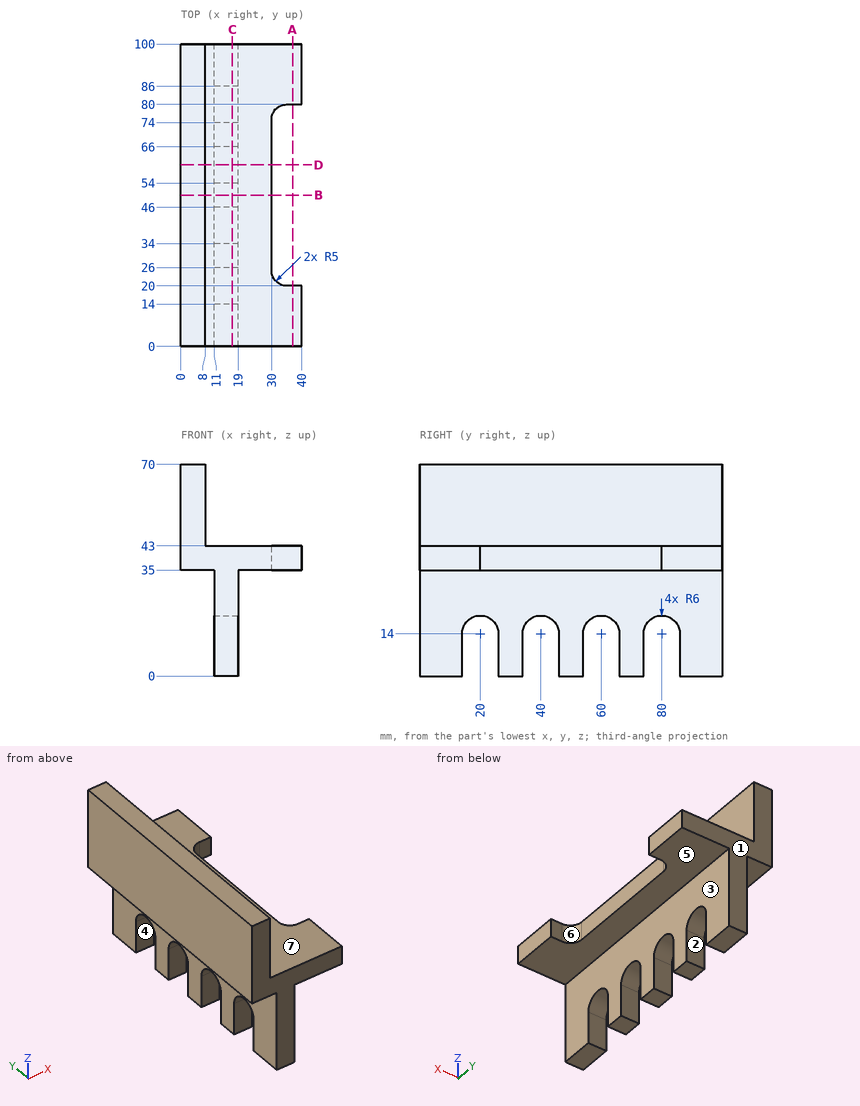
The figure shows three views and two pictorial views of one solid part (mm, origin at its lowest corner). Answer the questions. A direction names the side the tool comes from. Round coordinates to 2 decimals unless told otherwise and drop trailing zeros. Loops run counter-clockwise (first coordinate to the right, second up) from the corner with the lowest first, then second, coordinate; pieces in that order, holes last. Notation, with made-up numbers: M 24.5,27.5 L 38.5,27.5 A17 cw 38.5,48.5 Z; hole C 18.25,-15.5 d11. An arc over 180 degrees is marked long. Use CSV: the item, a comma, the result in double quotes.
Q1. The mould has two halves that part along Y. Classify the marked faces 1, 2 and 3: pulls with the +Y half, pulls with the -Y half, needs draft (parallel to the pull), parting line crosses it, or undercut.
Determined:
face 1,"pulls with the +Y half"
face 2,"undercut"
face 3,"needs draft"
Q2. Each of these flat-tipped pins is pushed along its axis until it touches: pin 1 (1 mm diameter, centred on x = 29.5, z = 42, fed in from -Y); pin 2 (8 mm diameter, centred on x = 24.5, y = 56.5, fed in from +Z); pin 3 (2.5 mm diameter, centred on y = 42.5, z = 40, fed in from +X); pin 4 (4 mm diameter, centred on y = 45, z = 49.5, fed in from +X). Where does it stop, or does it pass through?
Determined:
pin 1,"y = 0"
pin 2,"z = 43"
pin 3,"x = 30"
pin 4,"x = 8"
Q3. Section C-C, the plane x = 17 is taken. Determine the outline of the cut face in (y, z), then the cut area to 3 significant figures.
Determined:
outline,"M 0,0 L 14,0 L 14,14 A6 cw 26,14 L 26,0 L 34,0 L 34,14 A6 cw 46,14 L 46,0 L 54,0 L 54,14 A6 cw 66,14 L 66,0 L 74,0 L 74,14 A6 cw 86,14 L 86,0 L 100,0 L 100,43 L 0,43 Z"
area,"3,400 mm2"
Q4. A tool of negligible diameter and unlimited length cuts with its end or side. For the marked faces 4, 5, 6 and 7, from which of +Z, -Z, +X, -X, +Y, -Y can it reach the whole face along a straight path? Write none if from no direction.
Determined:
face 4,"-Z, +X, -X"
face 5,"-Z, +X, +Y, -Y"
face 6,"+Z, -Z, +X"
face 7,"+Z, +X, +Y, -Y"
Q5. Consider L1, parallel to Z at x = 2, y = 64; L2, parallel to Z at x = 36, y = 81; L3, parallel to X at y = 38, z = 56.5. Determine where each line is inside the solid, lowest interval first.
Determined:
L1,"35 to 70"
L2,"35 to 43"
L3,"0 to 8"
Q6. Section B-B, the plane y = 50 is taken. Determine the outline of the cut face in (x, z), then the cut area to 3 significant figures.
Determined:
outline,"M 0,35 L 11,35 L 11,0 L 19,0 L 19,35 L 30,35 L 30,43 L 8,43 L 8,70 L 0,70 Z"
area,"736 mm2"
Q7. Section A-A, the plane x = 37 is taken. Determine the outline of the cut face in (y, z).
Determined:
outline,"M 0,35 L 20,35 L 20,43 L 0,43 Z; M 80,35 L 100,35 L 100,43 L 80,43 Z"
Q8. Section D-D, the plane y = 60 is taken. Determine the outline of the cut face in (x, z), then the cut area to 3 significant figures.
Determined:
outline,"M 0,35 L 11,35 L 11,20 L 19,20 L 19,35 L 30,35 L 30,43 L 8,43 L 8,70 L 0,70 Z"
area,"576 mm2"
